Part model, mm, in its own coordinate system. A direction names the side the tool comes from. Give positions to 0.01 mm unless a question says otherwise; leave off trailing zeros. Order: outer loops, then holes, each group sorted by start corner. A loop starts at its lowest first (then second) coordinate and runs counter-clockwise, first axis right, second up. Notation, with made-up numbers: M 55,-36.5 L 86,-36.5 A13 cw 86,-31.5 Z; hole C 8.5,28 d6. An arc over 180 degrees is marked long. Return JSON: item names as keys, results as strings.
from build123d import *

# Parameters (mm, degrees)
BOSS_EXTRUDE1_DEPTH = 6.35
BOSS_EXTRUDE1_DRAFT = -1
CUT_EXTRUDE3_DEPTH  = 24.909662179
CIRPATTERN3_COUNT   = 24
BOSS_EXTRUDE3_DEPTH = 6.35
BOSS_EXTRUDE3_DRAFT = -1
SKETCH8_OUTSIDE_W   = 45.346
SKETCH8_OUTSIDE_H   = 42.089
CUT_EXTRUDE4_DEPTH  = 24.909662179
CUT_EXTRUDE4_DRAFT  = 5
DRAFT2_ANGLE        = -5
FILLET2_R           = 0.635


with BuildPart() as part:
    # Sketch1 → Boss-Extrude1 (with draft: the straight prism first)
    with BuildSketch(Plane(origin=(0, 0, 0), x_dir=(1, 0, 0), z_dir=(0, 1, 0))):
        with BuildLine():
            Line((-2.749630657, 15.625233333), (-14.906664335, -5.431366667))
            ThreePointArc((-14.906664335, -5.431366667), (-14.906664335, -8.606366667), (-12.157033678, -10.193866667))
            Line((-12.157033678, -10.193866667), (12.157033678, -10.193866667))
            ThreePointArc((12.157033678, -10.193866667), (14.906664335, -8.606366667), (14.906664335, -5.431366667))
            Line((14.906664335, -5.431366667), (2.749630657, 15.625233333))
            ThreePointArc((2.749630657, 15.625233333), (0, 17.212733333), (-2.749630657, 15.625233333))
        make_face()
    extrude(amount=-BOSS_EXTRUDE1_DEPTH)
    # Boss-Extrude1: the draft: its side faces are tilted about the plane it starts from
    boss_extrude1_sides = [part.faces().sort_by_distance(p)[0] for p in [
        (8.828147496, -3.175, -5.096933333),
        (0, -3.175, -17.212733333),
        (-8.828147496, -3.175, -5.096933333),
        (-14.906664335, -3.175, 8.606366667),
        (0, -3.175, 10.193866667),
        (14.906664335, -3.175, 8.606366667),
    ]]
    draft(boss_extrude1_sides, Plane(origin=(0, 0, 0), x_dir=(1, 0, 0), z_dir=(0, 1, 0)), BOSS_EXTRUDE1_DRAFT)

    # Sketch6 → Cut-Extrude3 (cut, through all)
    with BuildSketch(Plane.XY):
        Polygon((0, -2.54), (-6.985, -9.525), (6.985, -9.525), align=None)
    cut_extrude3 = extrude(amount=-CUT_EXTRUDE3_DEPTH, mode=Mode.SUBTRACT)

    # CirPattern3: Cut-Extrude3 ×24 about axis
    cirpattern3_axis = Axis((0, 0, 0), (0, 1, 0))
    for i in range(1, CIRPATTERN3_COUNT):
        add(cut_extrude3.rotate(cirpattern3_axis, i * 360 / CIRPATTERN3_COUNT), mode=Mode.SUBTRACT)


with BuildPart() as boss_extrude3_tool:
    # Sketch7 → Boss-Extrude3 (with draft: the straight prism first)
    with BuildSketch(Plane(origin=(0, 0, 0), x_dir=(1, 0, 0), z_dir=(0, 1, 0))):
        with BuildLine():
            Line((-12.157033678, -10.193866667), (12.157033678, -10.193866667))
            ThreePointArc((12.157033678, -10.193866667), (14.906664335, -8.606366667), (14.906664335, -5.431366667))
            Line((14.906664335, -5.431366667), (2.749630657, 15.625233333))
            ThreePointArc((2.749630657, 15.625233333), (0, 17.212733333), (-2.749630657, 15.625233333))
            Line((-2.749630657, 15.625233333), (-14.906664335, -5.431366667))
            ThreePointArc((-14.906664335, -5.431366667), (-14.906664335, -8.606366667), (-12.157033678, -10.193866667))
        make_face()
        with BuildLine():
            Line((-12.157033678, -8.034866667), (12.157033678, -8.034866667))
            ThreePointArc((12.157033678, -8.034866667), (13.036915488, -7.526866667), (13.036915488, -6.510866667))
            Line((13.036915488, -6.510866667), (0.87988181, 14.545733333))
            ThreePointArc((0.87988181, 14.545733333), (0, 15.053733333), (-0.87988181, 14.545733333))
            Line((-0.87988181, 14.545733333), (-13.036915488, -6.510866667))
            ThreePointArc((-13.036915488, -6.510866667), (-13.036915488, -7.526866667), (-12.157033678, -8.034866667))
        make_face(mode=Mode.SUBTRACT)
    extrude(amount=-BOSS_EXTRUDE3_DEPTH)
    # Boss-Extrude3: the draft: its side faces are tilted about the plane it starts from
    boss_extrude3_sides = [boss_extrude3_tool.faces().sort_by_distance(p)[0] for p in [
        (0, -3.175, 10.193866667),
        (14.906664335, -3.175, 8.606366667),
        (8.828147496, -3.175, -5.096933333),
        (0, -3.175, -17.212733333),
        (-8.828147496, -3.175, -5.096933333),
        (-14.906664335, -3.175, 8.606366667),
        (-13.036915488, -3.175, 7.526866667),
        (-6.958398649, -3.175, -4.017433333),
        (0, -3.175, -15.053733333),
        (6.958398649, -3.175, -4.017433333),
        (13.036915488, -3.175, 7.526866667),
        (0, -3.175, 8.034866667),
    ]]
    draft(boss_extrude3_sides, Plane(origin=(0, 0, 0), x_dir=(1, 0, 0), z_dir=(0, 1, 0)), BOSS_EXTRUDE3_DRAFT)


with BuildPart() as part_1:
    add(part.part)

    # Boss-Extrude3: add boss_extrude3_tool
    add(boss_extrude3_tool.part)


with BuildPart() as cut_extrude4_tool:
    # Sketch8 outside → Cut-Extrude4 (with draft: the straight prism first)
    with BuildSketch(Plane(origin=(0, 0, 0), x_dir=(1, 0, 0), z_dir=(0, 1, 0))):
        with Locations((0, 3.5095)):
            Rectangle(SKETCH8_OUTSIDE_W, SKETCH8_OUTSIDE_H)
        with BuildLine():
            Line((-12.157033678, -10.397066667), (12.157033678, -10.397066667))
            ThreePointArc((12.157033678, -10.397066667), (15.082640697, -8.707966667), (15.082640697, -5.329766667))
            Line((15.082640697, -5.329766667), (2.925607019, 15.726833333))
            ThreePointArc((2.925607019, 15.726833333), (0, 17.415933333), (-2.925607019, 15.726833333))
            Line((-2.925607019, 15.726833333), (-15.082640697, -5.329766667))
            ThreePointArc((-15.082640697, -5.329766667), (-15.082640697, -8.707966667), (-12.157033678, -10.397066667))
        make_face(mode=Mode.SUBTRACT)
    extrude(amount=-CUT_EXTRUDE4_DEPTH)
    # Cut-Extrude4: the draft: its side faces are tilted about the plane it starts from
    cut_extrude4_sides = [cut_extrude4_tool.faces().sort_by_distance(p)[0] for p in [
        (0, -12.45483109, 17.535),
        (22.673, -12.45483109, -3.5095),
        (0, -12.45483109, -24.554),
        (-22.673, -12.45483109, -3.5095),
        (-9.004123858, -12.45483109, -5.198533333),
        (0, -12.45483109, -17.415933333),
        (9.004123858, -12.45483109, -5.198533333),
        (15.082640697, -12.45483109, 8.707966667),
        (0, -12.45483109, 10.397066667),
        (-15.082640697, -12.45483109, 8.707966667),
    ]]
    draft(cut_extrude4_sides, Plane(origin=(0, 0, 0), x_dir=(1, 0, 0), z_dir=(0, 1, 0)), CUT_EXTRUDE4_DRAFT)


with BuildPart() as part_2:
    add(part_1.part)

    # Cut-Extrude4: cut by cut_extrude4_tool
    add(cut_extrude4_tool.part, mode=Mode.SUBTRACT)

    # Draft2
    draft2_faces = [part_2.faces().sort_by_distance(p)[0] for p in [
        (-13.104108463, -4.445, 7.565660548),
        (-7.03077319, -4.787774892, -4.059218794),
        (0, -4.445, -15.131321097),
        (7.03077319, -4.787774892, -4.059218794),
        (13.104108463, -4.445, 7.565660548),
        (0, -4.787774892, 8.118437588),
    ]]
    draft(draft2_faces, Plane(origin=(-12.157033678, 0, 7.018866667), x_dir=(0, 0, 1), z_dir=(0, 1, 0)), DRAFT2_ANGLE)

    # Fillet2
    fillet2_edges = [part_2.edges().sort_by_distance(p)[0] for p in [
        (-7.439521672, -6.35, -4.29520984),
        (-13.518038511, -6.35, 7.804643173),
        (0, -6.35, 8.59041968),
        (13.518038511, -6.35, 7.804643173),
        (7.439521672, -6.35, -4.29520984),
        (0, -6.35, -15.609286347),
        (-8.523000835, -6.35, -4.920756827),
        (-14.601517675, -6.35, 8.43019016),
        (0, -6.35, 9.841513653),
        (14.601517675, -6.35, 8.43019016),
        (8.523000835, -6.35, -4.920756827),
        (0, -6.35, -16.86038032),
    ]]
    fillet(fillet2_edges, radius=FILLET2_R)


solid = part_2.part
Q1. Two-plate mould, pull along X, no slides. Class faces 1 (the flat face through (-8.59, -4.32, -5.16)), 2 (the flat face through (6.91, -2.91, 1.47)), 3 (the flat face through (-0.31, -2.85, 5.97)), 4 (the conical face through (14.73, -4.32, 8.56)): +X half, -X half, draft (parallel to the pull), parting line (faces both ways), or undercut.
Established:
{"face 1": "-X half", "face 2": "undercut", "face 3": "undercut", "face 4": "+X half"}
Q2. 3-axis set-ups, long thin cutter, end or side, ignore diameter. For faces 5 (the cylindrical face through (8.31, -6.18, -4.99)), 6 (the flat face through (-2.186, -2.913, -6.717)): which of +Z, -Z, +X, -X, +Y, -Y reach the whole face in a straight line?
Established:
{"face 5": "-Z, +X, -Y", "face 6": "-Y"}
Q3. Band-saw the part on B-B (y = -1.75). Give the cut face in (x, z), then the cut area to 3 significant figures.
Established:
{"outline": "M -14.88,5.45 L -2.72,-15.61 A3.14 ccw 2.72,-15.61 L 14.88,5.45 A3.14 ccw 12.16,10.16 L -12.16,10.16 A3.14 ccw Z", "area": "516 mm²"}
Q4. Band-saw the part on A-A (y = -5). Give the cut face in (x, z), then the cut area to 3 significant figures.
Established:
{"outline": "M -14.7,5.55 L -2.55,-15.51 A2.94 ccw 2.55,-15.51 L 14.7,5.55 A2.94 ccw 12.16,9.96 L -12.16,9.96 A2.94 ccw Z; hole M -13.42,6.29 L -1.26,-14.76 A1.45 ccw 1.26,-14.76 L 13.42,6.29 A1.45 ccw 12.16,8.47 L -12.16,8.47 A1.45 ccw Z", "area": "129 mm²"}
Q5. Probe line 1 along X through (y, z) = (-3, -11.25); line 2 along X through (y, z) = (-4, 8); line 3 along Y through (x, z) = (12.5, 5). List the from-to ranges inside material, lowest first.
Established:
{"line 1": "x = -5.21 to -3.09, -2.54 to -0.46, 0.46 to 2.54, 3.09 to 5.21", "line 2": "x = -15.02 to -13.11, -10.94 to -10.06, 10.06 to 10.94, 13.11 to 15.02", "line 3": "y = -4.13 to 0"}
Q6. Pin check, flat tips, straight feed: pin 1 (1 mm diameter, centred on x = 10.5, y = -1.5, fed in from +Z); pin 2 (1 mm diameter, centred on y = -5.5, z = 6, fed in from +X); pin 3 (2 mm diameter, centred on x = -6, y = -4, fed in from +Z). Stop position of each tip, or through.
Established:
{"pin 1": "stops at z = 10.18", "pin 2": "stops at x = 15.02", "pin 3": "stops at z = 10.13"}
